Here's the drawing with two shaded views (mm, measured from the low corner). I have some questions. Round coordinates to 2 decimals unless told otherwise and drop trailing zeros. Loops run counter-clockwise (first coordinate to the right, second up) from the corner with the lowest first, then second, coordinate; pieces in that order, holes last.
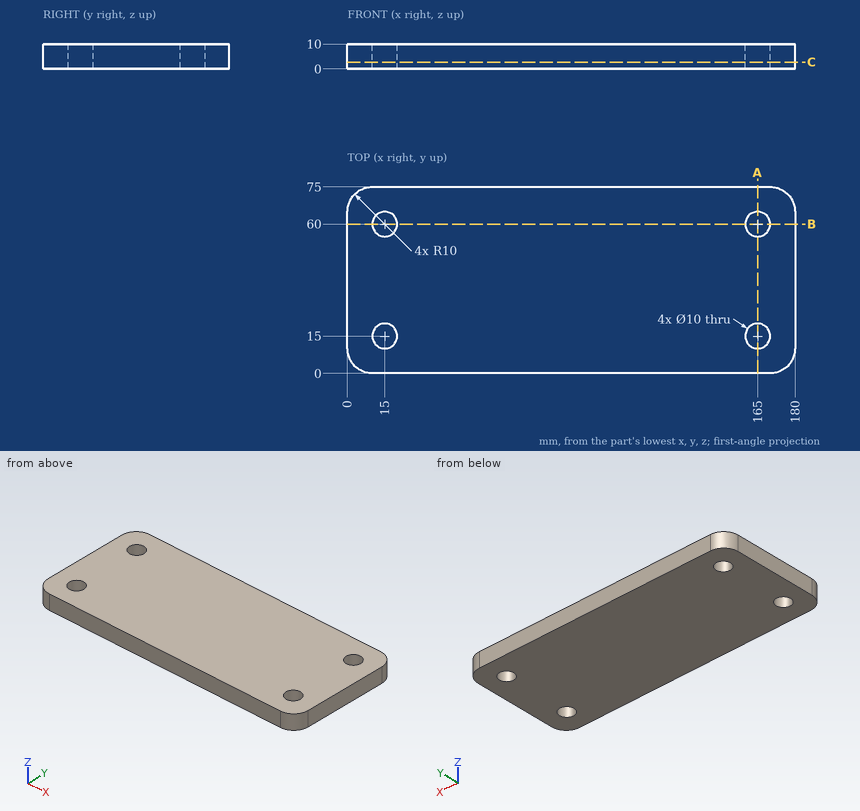
(1) If we section it at B-B, the plane y = 60: List the corners of the cut face in (x, z) for me, then the cut area to 3 significant figures.
Worked answers:
outline: (0, 0) - (10, 0) - (10, 10) - (0, 10) - close; (20, 0) - (160, 0) - (160, 10) - (20, 10) - close; (170, 0) - (180, 0) - (180, 10) - (170, 10) - close
area: 1,600 mm2
(2) If I drill on line 1 (Y direction, x = 15, z = 3.25); line 2 (Y direction, x = 13, z = 1.5); line 3 (X direction, y = 14, z = 4.25), over which ranges is the centre line in solid material (lowest first)?
Worked answers:
line 1: y = 0 to 10, 20 to 55, 65 to 75
line 2: y = 0 to 10.42, 19.58 to 55.42, 64.58 to 75
line 3: x = 0 to 10.1, 19.9 to 160.1, 169.9 to 180
(3) If we section it at A-A, the plane x = 165: List the corners of the cut face in (y, z) for me, then the cut area to 3 significant figures.
Worked answers:
outline: (0, 0) - (10, 0) - (10, 10) - (0, 10) - close; (20, 0) - (55, 0) - (55, 10) - (20, 10) - close; (65, 0) - (75, 0) - (75, 10) - (65, 10) - close
area: 550 mm2
(4) If we section it at C-C, the plane z = 2.75: List the corners of the cut face in (x, y) for me.
Worked answers:
outline: (0, 10) arc R10 ccw to (10, 0) - (170, 0) arc R10 ccw to (180, 10) - (180, 65) arc R10 ccw to (170, 75) - (10, 75) arc R10 ccw to (0, 65) - close; hole circle Ø10 at (15, 15); hole circle Ø10 at (15, 60); hole circle Ø10 at (165, 15); hole circle Ø10 at (165, 60)
